Here's the drawing with two shaded views (mm, measured from the low corner). I have some questions. A direction names the side the tool comes from. Round coordinates to 2 decimals unless told otherwise and drop trailing zeros. Loops run counter-clockwise (first coordinate to the right, second up) from the corner with the lowest first, then second, coordinate; pieces in that order, holes last. Notation, with made-up numbers: (31.25, -39) - (65.25, -39) arc R13 ccw to (65.25, -30) - close; hole circle Ø7 at (-33.5, 47). An arc over 180 degrees is marked (long way). Answer as CSV lines item,"result".
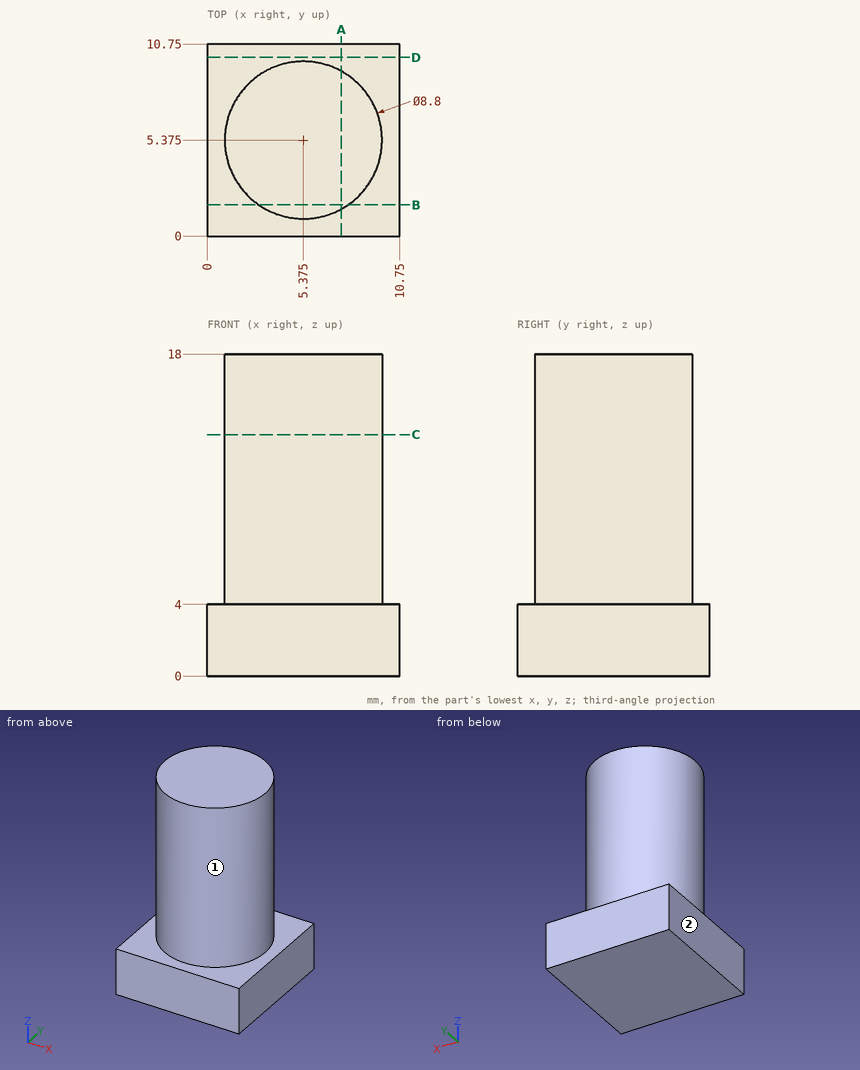
Q1. I'm going to push flat-ended pins straight in: pin 1 Ø6 at (y, z) = (4.5, 13.5) entering from -X (3 decimals); pin 2 Ø3 at (y, z) = (5, 6.5) entering from +X (3 decimals); pin 3 Ø1 at (y, z) = (9, 13) entering from -X; pin 4 Ø6 at (x, z) = (6, 6) entering from +Y. Where does each tip first touch, or does it pass through?
Checks:
pin 1,"x = 0.975"
pin 2,"x = 9.775"
pin 3,"x = 2.28"
pin 4,"y = 10.75"
Q2. Imagine slicing it at D-D (y = 10). Write out the boundary of the cut face in (x, z), then the cut area to 3 significant figures.
Checks:
outline,"(0, 0) - (10.75, 0) - (10.75, 4) - (0, 4) - close"
area,"43.0 mm²"
Q3. Imagine slicing it at C-C (z = 13.5). Write out the boundary of the cut face in (x, y) (3 decimals), then the cut area to 3 significant figures.
Checks:
outline,"circle Ø8.8 at (5.375, 5.375)"
area,"60.8 mm²"
Q4. Imagine slicing it at A-A (x = 7.5). Write out the boundary of the cut face in (y, z).
Checks:
outline,"(0, 0) - (10.75, 0) - (10.75, 4) - (9.23, 4) - (9.23, 18) - (1.52, 18) - (1.52, 4) - (0, 4) - close"
Q5. On a 3-axis mill with a long thin cutter (end or side, diameter ignored), from which of +Z, -Z, +X, -X, +Y, -Y can I reach the whole of each face in a straight line? I mean the marked faces 1 and 2. Say none if no direction works.
Checks:
face 1,"+Z"
face 2,"+Z, -Z, -X, +Y, -Y"
Q6. Imagine slicing it at B-B (y = 1.75). Write out the boundary of the cut face in (x, z), then the cut area to 3 significant figures.
Checks:
outline,"(0, 0) - (10.75, 0) - (10.75, 4) - (7.87, 4) - (7.87, 18) - (2.88, 18) - (2.88, 4) - (0, 4) - close"
area,"113 mm²"
Q7. If I drill on line 1 along Z through (x, y) = (4, 10); line 2 along X through (y, z) = (7.5, 16.5); line 3 along Y through (x, z) = (6.5, 6), over which ranges is the centre line in solid material (lowest first)? Write a range as [from, to].
Checks:
line 1,"[0, 4]"
line 2,"[1.52, 9.23]"
line 3,"[1.12, 9.63]"
